Source: CAD feature listing. Evaluate the final solid. Frame: model axes, mm. A direction names the side the tool comes from. Round coordinates to 2 decimals unless told otherwise and drop trailing zeros. Loops run counter-clockwise (first coordinate to the right, second up) from the corner with the lowest first, then second, coordinate; pieces in that order, holes last.
(1) First-contact query: pin 1 Ø3 at (x, z) = (0.53, 165.1) entering from -Y. Flat tip, straight axial feed; report the tip coordinate or a pass-through.
(2) Set-up query: faces 4 (the flat face through (1, 14.737, 128)), 5 (the flat face through (0, 16.007, 128)). Return all of +Z, -Z, +X, -X, +Y, -Y with unobstructed straight access to the full face (end or side cutting, diameter ignored); none if empty.
(3) Section A-A, the plane y = 8. Return the cut outline in (x, z), plus the area to 3 significant figures.
(4) Section C-C, the plane z = 178. Return the cut outline in (x, y), plus the area to 3 significant figures.
(5) Material intervals for probe 1 along Y at (x, z) = (-7, 127.5); probe 2 along X at (y, z) = (-34.2, 241.3); probe 3 along X at (y, z) = (8, 22), sorted ascending.
(6) Mould query, pull axis Z, two halves, no side actions, for faces 1 (the flat face through (1, -34.793, 128)), 2 (the cylindrical face through (-11.527, -14.865, 218.577)), 3 (the flat face through (-12, -9, 0)). Classes: pulls with the +Z half, pulls with the -Z half, needs draft (parallel to the pull), parting line crosses it, or undercut.
(7) Section D-D, the plane y = -14. Return the cut outline in (x, z), plus the area to 3 significant figures.
(8) Section B-B, the plane x = -5. Return the cut outline in (y, z).
Autodesk Inventor part; units mm, degrees
ref_plane "YZ Plane" through (0, 0, 0) normal (1, 0, 0) x (0, 1, 0)
ref_plane "XZ Plane" through (0, 0, 0) normal (0, 1, 0) x (-1, 0, 0)
ref_plane "XY Plane" through (0, 0, 0) normal (0, 0, 1) x (1, 0, 0)
sketch "Sketch1" plane through (0, 0, 0) normal (0, 0, 1) x (1, 0, 0)
  line L0 (-12.1708, 16.0073) -> (13.2292, 16.0073)
  line L1 (13.2292, 16.0073) -> (13.2292, -34.7927)
  line L2 (13.2292, -34.7927) -> (-12.1708, -34.7927)
  line L3 (-12.1708, -34.7927) -> (-12.1708, 16.0073)
  line L4 (11.9592, 14.7373) -> (-10.9008, 14.7373)
  line L5 (-10.9008, 14.7373) -> (-10.9008, -33.5227)
  line L6 (-10.9008, -33.5227) -> (11.9592, -33.5227)
  line L7 (11.9592, -33.5227) -> (11.9592, 14.7373)
  point P0 (0, 0)
  dimension "d0" = 25.4
  dimension "d1" = 50.8
  dimension "d2" = 1.27
extrude "Extrusion1" add sketch "Sketch1" along normal blind 260.35
sketch "Sketch2" plane through (-12.1708, 16.0073, 0) normal (0, 1, 0) x (1, 0, 0)
  circle A0 centre (12.7, -12.7) radius 1.7272
  line L0 (25.4, 0) -> (0, 0)
  line L1 (0, 0) -> (0, -260.35)
  point P0 (12.1708, 0)
  dimension "d5" = 3.4544
  dimension "d6" = 12.7
  dimension "d7" = 12.7
extrude "Extrusion2" cut sketch "Sketch2" against normal through all
pattern_linear "Rectangular Pattern1" count 26 spacing 25.4 along (0, 0, 1) of "Extrusion2"
sketch "Sketch5" plane through (13.2292, -34.7927, 0) normal (1, 0, 0) x (0, 0, -1)
  circle A0 centre (-231.775, 25.4) radius 14.2875
  line L0 (-260.35, 0) -> (-260.35, 50.8)
  line L1 (0, 50.8) -> (-260.35, 50.8)
  circle A1 centre (-28.575, 25.4) radius 14.2875
  line L2 (0, 0) -> (0, 50.8)
  point P0 (0, 34.7927)
  dimension "d46" = 28.575
  dimension "d48" = 25.4
  dimension "d52" = 28.575
  dimension "d54" = 25.4
  dimension "d62" = 28.575
  dimension "d63" = 28.575
extrude "Extrusion5" cut sketch "Sketch5" against normal through all
equation "\"d3\" = d13"
equation "\"d10\" = d14"
equation "\"d13\" = 260.35"
equation "\"d14\" = d13"
equation "\"d32\" = 101.6"
properties part number "AIntakeArm1"
Output values:
1. pin 1: passes through
2. face 4: +Z, -Z
2. face 5: +Z, -Z, +X, -X, +Y
3. outline: (-12.17, 0) - (-10.9, 0) - (-10.9, 260.35) - (-12.17, 260.35) - close; (11.96, 0) - (13.23, 0) - (13.23, 260.35) - (11.96, 260.35) - close
3. area: 661 mm2
4. outline: (-12.17, -34.79) - (13.23, -34.79) - (13.23, 16.01) - (-12.17, 16.01) - close; hole (-10.9, -33.52) - (11.96, -33.52) - (11.96, 14.74) - (-10.9, 14.74) - close
4. area: 187 mm2
5. probe 1: y = -34.79 to -33.52, 14.74 to 16.01
5. probe 2: x = -12.17 to -1.2, 2.26 to 13.23
5. probe 3: x = -12.17 to -10.9, 11.96 to 13.23
6. face 1: needs draft
6. face 2: undercut
6. face 3: pulls with the -Z half
7. outline: (-12.17, 0) - (-10.9, 0) - (-10.9, 15.05) - (-12.17, 15.05) - close; (-12.17, 42.1) - (-10.9, 42.1) - (-10.9, 218.25) - (-12.17, 218.25) - close; (-12.17, 245.3) - (-10.9, 245.3) - (-10.9, 260.35) - (-12.17, 260.35) - close; (11.96, 0) - (13.23, 0) - (13.23, 15.05) - (11.96, 15.05) - close; (11.96, 42.1) - (13.23, 42.1) - (13.23, 218.25) - (11.96, 218.25) - close; (11.96, 245.3) - (13.23, 245.3) - (13.23, 260.35) - (11.96, 260.35) - close
7. area: 524 mm2
8. outline: (-34.79, 0) - (-33.52, 0) - (-33.52, 260.35) - (-34.79, 260.35) - close; (14.74, 0) - (16.01, 0) - (16.01, 260.35) - (14.74, 260.35) - close
